Work out the finished part from the listing and answer in its coordinate system (mm). A direction names the side the tool comes from. Round coordinates to 2 decimals unless told otherwise and drop trailing zeros. Order: outer loops, then holes, each group sorted by start corner. A loop starts at its lowest first (then second) coordinate and runs counter-clockwise, first axis right, second up. Notation, with made-up numbers: M -32.75,86 L -2.75,86 A17 ccw -2.75,92 Z; hole C 67.5,59.25 d3. An arc over 180 degrees is marked long. Answer as a JSON object with one key per item and string values. Group by question number.
from build123d import *

# Parameters (mm, degrees)
SKETCH_1_R          = 2
EXTRUDE_1_DEPTH     = 1.5
SKETCH_2_W          = 9.5
SKETCH_2_H          = 9
EXTRUDE_2_DEPTH     = 3
SKETCH_3_W          = 6.5
SKETCH_3_H          = 9
CUT_EXTRUDE_1_DEPTH = 3
SKETCH_4_W          = 1.75
SKETCH_4_H          = 5
CUT_EXTRUDE_2_DEPTH = 3


with BuildPart() as part:
    # 草图1 → 凸台-拉伸1 (new body)
    with BuildSketch(Plane(origin=(0, 0, 0), x_dir=(1, 0, 0), z_dir=(0, 1, 0))):
        with BuildLine():
            Line((-4.75, 0), (-4.75, -14))
            Line((-4.75, -14), (4.75, -14))
            Line((4.75, -14), (4.75, 0))
            ThreePointArc((4.75, 0), (0, 4.75), (-4.75, 0))
        make_face()
        Circle(SKETCH_1_R, mode=Mode.SUBTRACT)
    extrude(amount=EXTRUDE_1_DEPTH)

    # 草图2 → 凸台-拉伸2 (add)
    with BuildSketch(Plane(origin=(0, 1.5, 0), x_dir=(1, 0, 0), z_dir=(0, 1, 0))):
        with Locations((0, -9.5)):
            Rectangle(SKETCH_2_W, SKETCH_2_H)
    extrude(amount=EXTRUDE_2_DEPTH)

    # 草图3 → 切除-拉伸1 (cut)
    with BuildSketch(Plane.XZ):
        with Locations((0, 9.5)):
            Rectangle(SKETCH_3_W, SKETCH_3_H)
    extrude(amount=-CUT_EXTRUDE_1_DEPTH, mode=Mode.SUBTRACT)

    # 草图4 → 切除-拉伸2 (cut)
    with BuildSketch(Plane(origin=(0, 4.5, 0), x_dir=(1, 0, 0), z_dir=(0, 1, 0))):
        with Locations((-3.875, -9.5)):
            Rectangle(SKETCH_4_W, SKETCH_4_H)
        with Locations((3.875, -9.5)):
            Rectangle(SKETCH_4_W, SKETCH_4_H)
    extrude(amount=-CUT_EXTRUDE_2_DEPTH, mode=Mode.SUBTRACT)


solid = part.part
Item 1: Find section D-D (z = -1.25). Give the vertices of the cut face in (x, y), and give its area (3 significant figures).
Item 2: Each of these flat-tipped pins is pushed along its axis until it touches: pin 1 (2 mm diameter, centred on y = 1.5, z = -1, fed in from -X); pin 2 (1.2 mm diameter, centred on y = 4, z = 10, fed in from +X); pin 3 (0.8 mm diameter, centred on x = -4, z = 9.5, fed in from +Y); pin 4 (0.8 mm diameter, centred on y = 3.5, z = 9.5, fed in from -X). Where does it stop, or does it pass through?
Item 3: Consider L1, parallel to X at y = 0.45, z = 0; L2, parallel to Z at x = 0, y = 1.1; L3, parallel to X at y = 0.75, z = 10.75. Determine where each line is inside the solid, lowest interval first.
Item 4: A tool of negligible diameter and unlimited length cuts with its end or side. For faces 4 (the flat face through (4, 1.5, 9)), 5 (the flat face through (0, 4, 5)), 6 (the flat face through (0, 1, 5)), from which of +Z, -Z, +X, -X, +Y, -Y can it reach the whole face along a straight path? Write none if from no direction.
Item 5: Find section A-A (x = 0). Give the vertices of the cut face in (y, z).
Item 6: Find section B-B (y = 1.1). Give the vertices of the cut face in (x, z).
Item 7: Find section C-C (z = 9.75). Give the vertices of the cut face in (x, y).
Item 8: The mould has two halves that part along X. Classify faces 1 (the flat face through (4.75, 1, 7)), 2 (the flat face through (-3.25, 1, 9)), 3 (the flat face through (4, 3, 7)): +X half, -X half, draft (parallel to the pull), parting line (faces both ways), or undercut.
Responses:
{
 "1": {"outline": "M -4.58,0 L -1.56,0 L -1.56,1.5 L -4.58,1.5 Z; M 1.56,0 L 4.58,0 L 4.58,1.5 L 1.56,1.5 Z", "area": "9.06 mm^2"},
 "2": {"pin 1": "stops at x = -4.75", "pin 2": "stops at x = 3", "pin 3": "stops at y = 1.5", "pin 4": "stops at x = -3"},
 "3": {"L1": "x = -4.75 to -2, 2 to 4.75", "L2": "z = -4.75 to -2, 2 to 5", "L3": "x = -4.75 to -3.25, 3.25 to 4.75"},
 "4": {"face 4": "+X, -X, +Y", "face 5": "-Z, +X, -X, +Y", "face 6": "+Z, -Y"},
 "5": {"outline": "M 0,-4.75 L 1.5,-4.75 L 1.5,-2 L 0,-2 Z; M 0,2 L 1.5,2 L 1.5,5 L 0,5 Z; M 3,5 L 4.5,5 L 4.5,14 L 3,14 Z"},
 "6": {"outline": "M -4.75,0 A4.75 ccw 4.75,0 L 4.75,14 L 3.25,14 L 3.25,5 L -3.25,5 L -3.25,14 L -4.75,14 Z; hole C 0,0 d4"},
 "7": {"outline": "M -4.75,0 L -3.25,0 L -3.25,1.5 L -4.75,1.5 Z; M -3,3 L 3,3 L 3,4.5 L -3,4.5 Z; M 3.25,0 L 4.75,0 L 4.75,1.5 L 3.25,1.5 Z"},
 "8": {"face 1": "+X half", "face 2": "undercut", "face 3": "draft"}
}
